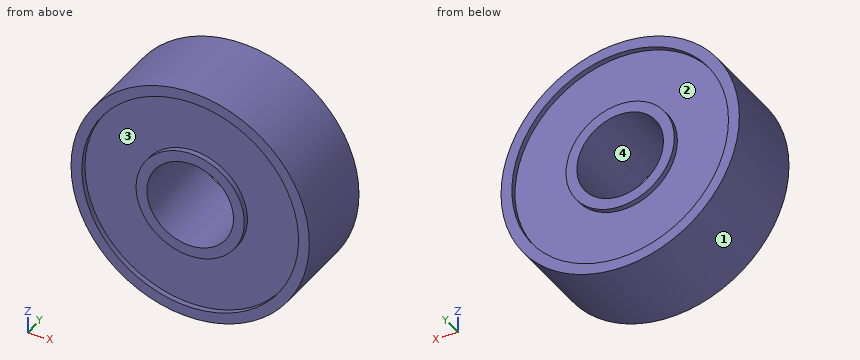
Autodesk Inventor part; units mm, degrees
ref_plane "YZ Plane" through (0, 0, 0) normal (1, 0, 0) x (0, 1, 0)
ref_plane "XZ Plane" through (0, 0, 0) normal (0, 1, 0) x (-1, 0, 0)
ref_plane "XY Plane" through (0, 0, 0) normal (0, 0, 1) x (1, 0, 0)
sketch "Sketch1" plane through (0, 0, 0) normal (0, 1, 0) x (-1, 0, 0)
  circle A0 centre (0, 0) radius 4
  circle A1 centre (0, 0) radius 5
  circle A2 centre (0, 0) radius 11
  circle A3 centre (0, 0) radius 10
  dimension "d0" = 8
  dimension "d1" = 10
  dimension "d2" = 22
  dimension "d3" = 20
extrude "Extrusion1" add sketch "Sketch1" along normal blind 7.5 contours A3
extrude "Extrusion2" add sketch "Sketch1" along normal blind 8 contours A2
extrude "Extrusion3" cut sketch "Sketch1" along normal blind 0.5 contours A3
extrude "Extrusion4" add sketch "Sketch1" along normal blind 8 contours A1
properties part number "bearing"
Part model, mm, in its own coordinate system. Face numbers are marked on the shaded views. A direction names the side the tool comes from. Give positions to 0.01 mm unless a question says otherwise; leave off trailing zeros. Loops run counter-clockwise (first coordinate to the right, second up) from the corner with the lowest first, then second, coordinate; pieces in that order, holes last. Notation, with made-up numbers: M 67,-28 L 95,-28 A34 cw 95,10 Z; hole C 2,16.25 d8. An arc over 180 degrees is marked long. Put each result on its own line as item: value. Start each with the question number.
1) Flat gauge pins, fed straight in: pin 1 (1 mm diameter, centred on y = 7, z = -8, fed in from -X); pin 2 (3 mm diameter, centred on y = 1, z = -8, fed in from +X); pin 3 (2 mm diameter, centred on x = 7, z = -0.5, fed in from -Y). Where does each tip first touch, or does it go through?
2) Saw through at D-D (z = -4.5). List the corners of the cut face in (x, y).
3) 3-axis set-ups, long thin cutter, end or side, ignore diameter. For the marked faces 3 and 4: which of +Z, -Z, +X, -X, +Y, -Y reach the whole face in a straight line?
4) Pull direction Z, two halves, no side cores. Call the marked faces 1 and 2: +Z half, -Z half, draft (parallel to the pull), parting line (faces both ways), or undercut.
5) Saw through at A-A (x = 0). List the corners of the cut face in (y, z), then the cut area to 3 significant figures.
6) Saw through at B-B (z = 0). List the corners of the cut face in (x, y), then the cut area to 3 significant figures.
7) Probe probe 1 along Z at (x, y) = (0, 0.35); probe 2 along Y at (x, z) = (9.75, 2); probe 3 along X at (y, z) = (7.75, 0.5). List the from-to ranges inside material, lowest first.
8) Saw through at C-C (y = 3). List the corners of the cut face in (x, z), then the cut area to 3 significant figures.
Numbers:
1. pin 1: x = -8.05
1. pin 2: x = 8.87
1. pin 3: y = 0.5
2. outline: M -10.04,0 L -8.93,0 L -8.93,0.5 L -2.18,0.5 L -2.18,0 L 2.18,0 L 2.18,0.5 L 8.93,0.5 L 8.93,0 L 10.04,0 L 10.04,8 L 8.93,8 L 8.93,7.5 L 2.18,7.5 L 2.18,8 L -2.18,8 L -2.18,7.5 L -8.93,7.5 L -8.93,8 L -10.04,8 Z
3. face 3: -Y
3. face 4: +Y, -Y
4. face 1: parting line
4. face 2: undercut
5. outline: M 0,-11 L 8,-11 L 8,-10 L 7.5,-10 L 7.5,-5 L 8,-5 L 8,-4 L 0,-4 L 0,-5 L 0.5,-5 L 0.5,-10 L 0,-10 Z; M 0,4 L 8,4 L 8,5 L 7.5,5 L 7.5,10 L 8,10 L 8,11 L 0,11 L 0,10 L 0.5,10 L 0.5,5 L 0,5 Z
5. area: 102 mm^2
6. outline: M -11,0 L -10,0 L -10,0.5 L -5,0.5 L -5,0 L -4,0 L -4,8 L -5,8 L -5,7.5 L -10,7.5 L -10,8 L -11,8 Z; M 4,0 L 5,0 L 5,0.5 L 10,0.5 L 10,0 L 11,0 L 11,8 L 10,8 L 10,7.5 L 5,7.5 L 5,8 L 4,8 Z
6. area: 102 mm^2
7. probe 1: -11 to -10, -5 to -4, 4 to 5, 10 to 11
7. probe 2: 0.5 to 7.5
7. probe 3: -10.99 to -9.99, -4.97 to -3.97, 3.97 to 4.97, 9.99 to 10.99
8. outline: C 0,0 d22; hole C 0,0 d8
8. area: 330 mm^2
